Can you work these out from the model? Positions are in its coordinate system, mm. Give positions to 0.01 mm unless a question says otherwise; leave off trailing zeros. Order: outer loops, then holes, each group sorted by start corner. A loop starts at its lowest first (then second) coordinate and runs counter-clockwise, first axis right, second up. Notation, with made-up numbers: (-13.75, 36.5) - (-0.75, 36.5) arc R14 cw to (-0.75, 48.5) - close; hole circle Ø7 at (-6.75, -38). An arc over 180 degrees is marked (long way). Return JSON: item names as keys, results as strings.
Autodesk Fusion 360 part; units mm, degrees
sketch "RectangleWithCircle" plane through (0, 0, 0) normal (0, 0, 1) x (1, 0, 0)
  line L0 (-38.1, -25.4) -> (38.1, -25.4)
  line L1 (38.1, -25.4) -> (38.1, 25.4)
  line L2 (38.1, 25.4) -> (-38.1, 25.4)
  line L3 (-38.1, 25.4) -> (-38.1, -25.4)
  circle A0 centre (0, 0) radius 12.7
  dimension "d1" = 76.2
  dimension "d2" = 50.8
  dimension "d3" = 25.4
sketch "Sketch2" plane through (0, 0, 0) normal (0, 0, 1) x (1, 0, 0)
  line L0 (-38.1, -25.4) -> (38.1, -25.4)
  line L1 (38.1, -25.4) -> (38.1, 25.4)
  line L2 (38.1, 25.4) -> (-38.1, 25.4)
  line L3 (-38.1, 25.4) -> (-38.1, -25.4)
  dimension "d6" = 50.8
  dimension "d7" = 76.2
extrude "Extrude1" add sketch "Sketch2" along normal blind 12.7
extrude "Extrude2" cut sketch "RectangleWithCircle" along normal through all contours A0
equation "d3 = ( 1.27 cm ) * 2"
1. If I drill on L1, parallel to X at y = 0, z = 7; L2, parallel to Y at x = 0, z = 10.25; L3, parallel to Y at x = 3.5, z = 7.5, over which ranges is the centre line in solid material (lowest first)? Write a range as [from, to].
Checks:
{"L1": "[-38.1, -12.7], [12.7, 38.1]", "L2": "[-25.4, -12.7], [12.7, 25.4]", "L3": "[-25.4, -12.21], [12.21, 25.4]"}
2. Suppose I cut it at C-C (z = 2.25). List the corners of the cut face in (x, y) for me.
Checks:
{"outline": "(-38.1, -25.4) - (38.1, -25.4) - (38.1, 25.4) - (-38.1, 25.4) - close; hole circle Ø25.4 at (0, 0)"}
3. Suppose I cut it at B-B (y = -10). List the corners of the cut face in (x, z) for me.
Checks:
{"outline": "(-38.1, 0) - (-7.83, 0) - (-7.83, 12.7) - (-38.1, 12.7) - close; (7.83, 0) - (38.1, 0) - (38.1, 12.7) - (7.83, 12.7) - close"}
4. Suppose I cut it at A-A (x = 0). List the corners of the cut face in (y, z) for me.
Checks:
{"outline": "(-25.4, 0) - (-12.7, 0) - (-12.7, 12.7) - (-25.4, 12.7) - close; (12.7, 0) - (25.4, 0) - (25.4, 12.7) - (12.7, 12.7) - close"}
5. Thinking about a two-plate mould opening in X: for faces 1 (the face through (8, 12, 0)), 2 (the face through (38.1, 0, 6)), 3 (the face through (-2.75, 12.4, 6.26)), which applies, +X half, -X half, draft (parallel to the pull), parting line (faces both ways), or undercut?
Checks:
{"face 1": "draft", "face 2": "+X half", "face 3": "undercut"}
